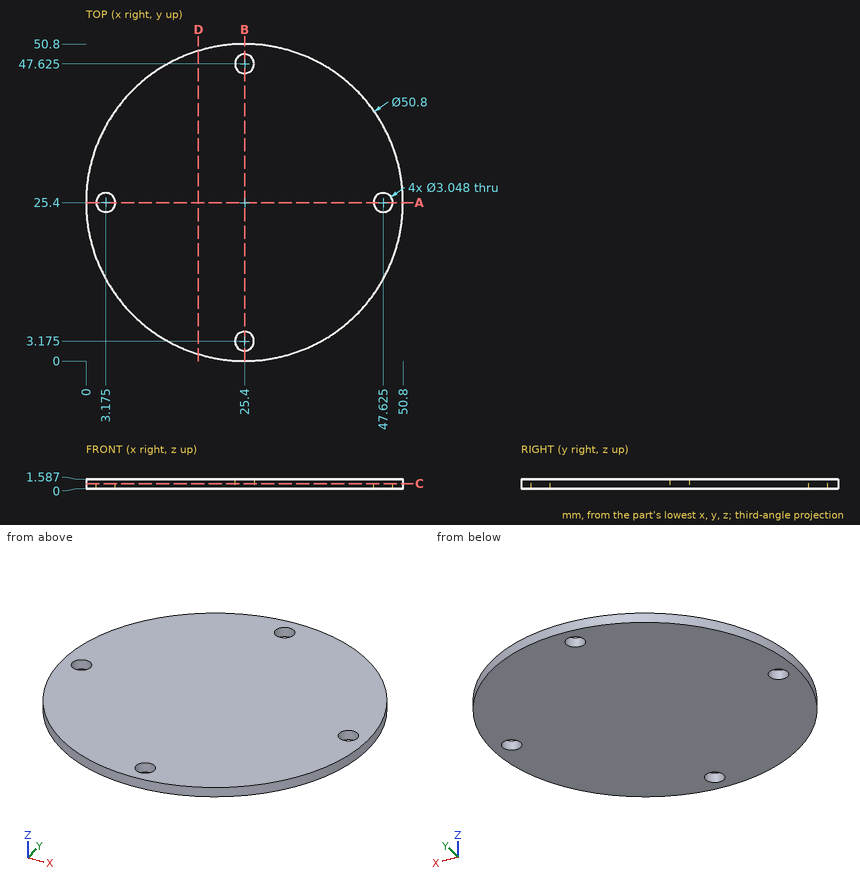
For this review, use the dimensioned drawing (mm, ordinates from the lowest corner) and the shaded views. Round coordinates to 2 decimals unless told otherwise and drop trailing zeros. Write each loop counter-clockwise with the first axis right and the second up, starting at its lowest first coordinate (ties: lowest second). Pieces come first, ordered by that corner, then holes. Notation, with made-up numbers: M 24,8.25 L 40,8.25 A32 cw 40,42.25 Z; hole C -17.75,-34.75 d1. An arc over 180 degrees is marked long. Answer as CSV lines item,"result". Start each with the question number.
Q1. Wall thickness on line 1 along Y through (x, z) = (25.4, 0.45); line 2 along Y through (x, z) = (4, 0.45) (1 decimal); line 3 along X through (y, z) = (3, 1.55) (1 decimal): over which ranges is each line inside the solid? List them lowest first.
Q2. Consider section C-C, the plane z = 0.85. Give the boundary of the cut face in (x, y) (1 decimal), then the cut area to 3 significant figures.
Q3. Consider section D-D, the plane x = 18. Give the boundary of the cut face in (y, z).
Q4. Consider section A-A, the plane y = 25.4. Give the boundary of the cut face in (x, z).
Result set:
1,line 1,"y = 0 to 1.65, 4.7 to 46.1, 49.15 to 50.8"
1,line 2,"y = 11.7 to 24.1, 26.7 to 39.1"
1,line 3,"x = 13.4 to 23.9, 26.9 to 37.4"
2,outline,"C 25.4,25.4 d50.8; hole C 3.2,25.4 d3; hole C 25.4,3.2 d3; hole C 25.4,47.6 d3; hole C 47.6,25.4 d3"
2,area,"2,000 mm²"
3,outline,"M 1.1,0 L 49.7,0 L 49.7,1.59 L 1.1,1.59 Z"
4,outline,"M 0,0 L 1.65,0 L 1.65,1.59 L 0,1.59 Z; M 4.7,0 L 46.1,0 L 46.1,1.59 L 4.7,1.59 Z; M 49.15,0 L 50.8,0 L 50.8,1.59 L 49.15,1.59 Z"
